Can you work these out from the model? Positions are in its coordinate system, mm. A direction names the side the tool comes from. Give positions to 0.01 mm unless a question says otherwise; leave off trailing zeros. Write each loop counter-clockwise with the first axis right and the second up, starting at its lowest first coordinate (ties: lowest second). Pieces come first, ordered by that corner, then holes.
Autodesk Inventor part; units mm, degrees
ref_plane "YZ Plane" through (0, 0, 0) normal (1, 0, 0) x (0, 1, 0)
ref_plane "XZ Plane" through (0, 0, 0) normal (0, 1, 0) x (-1, 0, 0)
ref_plane "XY Plane" through (0, 0, 0) normal (0, 0, 1) x (1, 0, 0)
sketch "Sketch1" plane through (0, 0, 0) normal (0, 1, 0) x (-1, 0, 0)
  circle A0 centre (0, 0) radius 45
  circle A1 centre (0, 0) radius 25.5
  dimension "d0" = 90
  dimension "d1" = 51
extrude "Extrusion1" add sketch "Sketch1" along normal blind 40
sketch "Sketch2" plane through (0, 0, 0) normal (0, -1, 0) x (1, 0, 0)
  circle A0 centre (0, 0) radius 25.5
  circle A1 centre (0, 0) radius 45
  line L0 (6.2, 0) -> (3.1, -5.3694)
  line L1 (3.1, -5.3694) -> (-3.1, -5.3694)
  line L2 (-3.1, -5.3694) -> (-6.2, 0)
  line L3 (-6.2, 0) -> (-3.1, 5.3694)
  line L4 (-3.1, 5.3694) -> (3.1, 5.3694)
  line L5 (3.1, 5.3694) -> (6.2, 0)
  line L6 (-3.1, 5.3694) -> (-3.1, 25.3109)
  line L7 (3.1, 5.3694) -> (3.1, 25.3109)
  line L8 (6.2, 0) -> (23.4699, -9.9708)
  line L9 (3.1, -5.3694) -> (20.3699, -15.3401)
  line L10 (-3.1, -5.3694) -> (-20.3699, -15.3401)
  line L11 (-6.2, 0) -> (-23.4699, -9.9708)
  circle A2 centre (0, 0) radius 6.5
  dimension "d4" = 6.2
  dimension "d5" = 13
extrude "Extrusion2" add sketch "Sketch2" against normal blind 15 contours L7 A2 L6 A0 | A0 L9 A2 L8 | A2 L8 L5 L7 | L7 L4 L6 A2 | A2 L9 L0 L8 | L11 A2 L10 A0 | L6 L3 L11 A2 | A2 L10 L1 L9 | L11 L2 L10 A2
sketch "Sketch3" plane through (0, 0, 0) normal (0, -1, 0) x (1, 0, 0)
  line L0 (3.1, -5.3694) -> (-3.1, -5.3694)
  line L1 (-3.1, -5.3694) -> (-6.2, 0)
  line L2 (-6.2, 0) -> (-3.1, 5.3694)
  line L3 (-3.1, 5.3694) -> (3.1, 5.3694)
  line L4 (3.1, 5.3694) -> (6.2, 0)
  line L5 (6.2, 0) -> (3.1, -5.3694)
  circle A0 centre (0, 0) radius 45
  circle A1 centre (0, 0) radius 2
  dimension "d8" = 4
extrude "Extrusion3" add sketch "Sketch3" against normal blind 5 contours L0 L1 L2 L3 L4 L5
properties part number "koleso" material "ABS Plastic"
1) If we mould it in two halves opening along X, with no side actions, what happens to faces 3 (the face through (-1, 0, 11)), 4 (the face through (-11.76, 7.4, -10.37)), 5 (the face through (-20.765, 19.72, 39.923))? For each: +X half, -X half, draft (parallel to the pull), parting line (faces both ways), or undercut.
Values follow:
face 3: draft
face 4: undercut
face 5: parting line
2) For faces 1 (the face through (4.63, 9.93, 2.72)), 2 (the face through (3.1, 7, 15)), which set-ups out of +Z, -Z, +X, -X, +Y, -Y let a thin tool reach every point of the face, with its end or its side?
Values follow:
face 1: +Y
face 2: +Y, -Y
3) Suppose I cut it at B-B on z = 22. Write out the boundary of the cut face in (x, y), plus the area to 3 significant figures.
Values follow:
outline: (-39.26, 0) - (-12.89, 0) - (-12.89, 40) - (-39.26, 40) - close; (-3.1, 0) - (3.1, 0) - (3.1, 15) - (-3.1, 15) - close; (12.89, 0) - (39.26, 0) - (39.26, 40) - (12.89, 40) - close
area: 2,200 mm2
4) Suppose I cut it at C-C on z = -23.5. Write out the boundary of the cut face in (x, y).
Values follow:
outline: (-38.38, 0) - (-9.9, 0) - (-9.9, 40) - (-38.38, 40) - close; (9.9, 0) - (38.38, 0) - (38.38, 40) - (9.9, 40) - close
5) Suppose I cut it at A-A on x = 0. Write out the boundary of the cut face in (y, z).
Values follow:
outline: (0, -45) - (40, -45) - (40, -25.5) - (0, -25.5) - close; (0, -6.5) - (15, -6.5) - (15, -5.37) - (5, -5.37) - (5, -2) - (0, -2) - close; (0, 2) - (5, 2) - (5, 5.37) - (15, 5.37) - (15, 25.5) - (40, 25.5) - (40, 45) - (0, 45) - close
6) For pin 1 Ø10 at (y, z) = (16.5, 29) entering from +X; pin 2 Ø3 at (x, y) = (1, 8.5) entering from +Z; pin 3 Ø8.5 at (x, z) = (2, -2.5) entering from +Y; pin 4 Ø3 at (x, z) = (0, 0) entering from -Y (3 decimals), each with a flat end and sliding along its axis, tell me the tip position at first contact or that it passes through.
Values follow:
pin 1: stops at x = 38.07
pin 2: stops at z = 45
pin 3: stops at y = 15
pin 4: passes through
7) Please list where these lines run through material, in increasing order: L1, parallel to Z at x = 0, y = 3.3; L2, parallel to Z at x = 0, y = 8; L3, parallel to X at y = 17, z = 0.5.
Values follow:
L1: z = -45 to -25.5, -6.5 to -2, 2 to 45
L2: z = -45 to -25.5, -6.5 to -5.37, 5.37 to 45
L3: x = -45 to -25.5, 25.5 to 45
8) Suppose I cut it at D-D on y = 35.5. Write out the boundary of the cut face in (x, z), plus the area to 3 significant figures.
Values follow:
outline: circle Ø90 at (0, 0); hole circle Ø51 at (0, 0)
area: 4,320 mm2
